from build123d import *

# Parameters (mm, degrees)
BOSS_EXTRUDE1_DEPTH = 50
SKETCH2_R           = 1.5
BOSS_EXTRUDE2_DEPTH = 2
CUT_EXTRUDE1_DEPTH  = 6


with BuildPart() as part:
    # Sketch1 → Boss-Extrude1 (new body)
    with BuildSketch(Plane.XY):
        Polygon((5, 36), (0, 38), (0, 0), (5, 2), align=None)
    extrude(amount=BOSS_EXTRUDE1_DEPTH)

    # Sketch2 → Boss-Extrude2 (add)
    with BuildSketch(Plane(origin=(5, 0, 0), x_dir=(0, 0, -1), z_dir=(1, 0, 0))):
        with BuildLine():
            Line((-50, 13), (-54, 13))
            ThreePointArc((-54, 13), (-57, 16), (-54, 19))
            Line((-54, 19), (-50, 19))
            ThreePointArc((-50, 19), (-47, 16), (-50, 13))
        make_face()
        with Locations((-54, 16)):
            Circle(SKETCH2_R, mode=Mode.SUBTRACT)
    extrude(amount=-BOSS_EXTRUDE2_DEPTH)

    # Sketch3 → Cut-Extrude1 (cut, through all)
    with BuildSketch(Plane(origin=(5, 0, 0), x_dir=(0, 0, -1), z_dir=(1, 0, 0))):
        with BuildLine():
            Line((-36.547631245, 31.375), (-14.547631245, 8.137099923))
            ThreePointArc((-14.547631245, 8.137099923), (-14.625, 5.309731168), (-17.452368755, 5.387099923))
            Line((-17.452368755, 5.387099923), (-39.452368755, 28.625))
            ThreePointArc((-39.452368755, 28.625), (-39.375, 31.452368755), (-36.547631245, 31.375))
        make_face()
    extrude(amount=-CUT_EXTRUDE1_DEPTH, mode=Mode.SUBTRACT)


solid = part.part
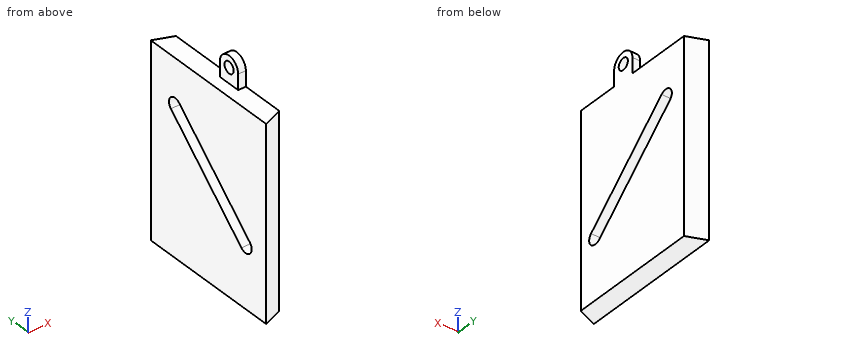
CAD build for the part. Positions are in the model's coordinates, mm. Coordinates: 2 decimals unless noted, no trailing zeros. Loops run counter-clockwise (first coordinate to the right, second up) from the corner with the lowest first, then second, coordinate; pieces in that order, holes last. Notation, with made-up numbers: (5.5, 9) -> (38.5, 9) arc R22 ccw to (38.5, 41) -> close; hole circle Ø3 at (20, 78). An arc over 180 degrees is marked (long way). One line per item, written item: value.
1. Flat gauge pins, fed straight in: P1, Ø1, axis at x = 4.5, z = 51.5, coming from the +Y side; P2, Ø2.5, axis at y = 16, z = 54, coming from the -X side; P3, Ø1.6, axis at x = 3.5, z = 52.5, coming from the -Y side; P4, Ø1.5, axis at x = 3, y = 20, coming from the +Z side. Where does each tip first touch, or does it go through?
Answers:
P1: stops at y = 19
P2: passes through
P3: stops at y = 13
P4: stops at z = 50
2. Slice it at B-B on y = 30. Write the cut outline in (x, z), and give its area (3 significant figures).
Answers:
outline: (0, 0) -> (5, 0) -> (5, 35.25) -> (0, 35.25) -> close; (0, 40) -> (5, 40) -> (5, 50) -> (0, 50) -> close
area: 226 mm^2
3. Drill centre lines: line 1 (Y direction, x = 4.5, z = 54); line 2 (Z direction, x = 3, y = 21); line 3 (Z direction, x = 2.8, y = 2). Where is each one in solid material? Low to high. Write a range as [from, to].
Answers:
line 1: y = [13, 14.5], [17.5, 19]
line 2: z = [0, 26.73], [32.23, 50]
line 3: z = [0, 50]
4. Slice it at A-A on z = 26. Write the cut outline in (x, y).
Answers:
outline: (0, 0) -> (5, 2) -> (5, 14.42) -> (0, 14.42) -> close; (0, 20.23) -> (5, 20.23) -> (5, 36) -> (0, 38) -> close
5. Slice it at D-D on y = 16. Write the cut outline in (x, z).
Answers:
outline: (0, 0) -> (5, 0) -> (5, 21.99) -> (0, 21.99) -> close; (0, 27.5) -> (5, 27.5) -> (5, 52.5) -> (3, 52.5) -> (3, 50) -> (0, 50) -> close; (3, 55.5) -> (5, 55.5) -> (5, 57) -> (3, 57) -> close
6. Slice it at C-C on x = 0.7. Write the cut outline in (y, z) (3 decimals).
Answers:
outline: (0.28, 0) -> (37.72, 0) -> (37.72, 50) -> (0.28, 50) -> close; hole (5.387, 17.452) arc R2 ccw to (8.137, 14.548) -> (31.375, 36.548) arc R2 ccw to (28.625, 39.452) -> close
